Part model, mm, in its own coordinate system. Coordinates: 2 decimals unless noted, no trailing zeros. Order: outer loops, then holes, each group sorted by start corner. A loop starts at its lowest first (then second) coordinate and runs counter-clockwise, first axis right, second up. Notation, with made-up numbers: M -32.5,64 L -7.5,64 A6 ccw -7.5,73 Z; hole C 64,70.25 d4. An arc over 180 degrees is marked long. Answer in a Markdown table with one row per item. Add a question column.
from build123d import *

# Parameters (mm, degrees)
FILLET1_R          = 2.54
SKETCH2_R          = 1.395150395
CUT_EXTRUDE1_DEPTH = 126.080494205


with BuildPart() as part:
    # Sketch1 → Revolve1 (revolve)
    with BuildSketch(Plane.XY, mode=Mode.PRIVATE) as revolve1_sk:
        with BuildLine():
            Line((0, 76.2), (6.35, 76.2))
            Line((6.35, 76.2), (6.35, 63.5))
            ThreePointArc((6.35, 63.5), (51.251280605, 44.901280605), (69.85, 0))
            Line((69.85, 0), (63.5, 0))
            ThreePointArc((63.5, 0), (46.761152545, 40.411152545), (6.35, 57.15))
            Line((6.35, 57.15), (0, 57.15))
            Line((0, 57.15), (0, 76.2))
        make_face()
    revolve(revolve1_sk.sketch.rotate(Axis((0, 0, 0), (1, 0, 0)), 90), axis=Axis((0, 0, 0), (1, 0, 0)))

    # Fillet1
    fillet1_edges = [part.edges().sort_by_distance(p)[0] for p in [
        (6.35, 0, -63.5),
    ]]
    fillet(fillet1_edges, radius=FILLET1_R)

    # Sketch2 → Cut-Extrude1 (cut, through all)
    with BuildSketch(Plane(origin=(6.35, 0, 0), x_dir=(0, 0, -1), z_dir=(1, 0, 0))):
        with Locations((0, 73.025)):
            Circle(SKETCH2_R)
        with Locations((73.025, 0)):
            Circle(SKETCH2_R)
        with Locations((0, -73.025)):
            Circle(SKETCH2_R)
        with Locations((-73.025, 0)):
            Circle(SKETCH2_R)
    extrude(amount=-CUT_EXTRUDE1_DEPTH, mode=Mode.SUBTRACT)


solid = part.part
(1) Slice it at A-A (x = 57). List the corners of the cut face in (y, z).
(2) Wall check: line 1 (Y direction, x = 2.5, z = 0); line 2 (Y direction, x = 9.5, z = 42); line 3 (Y direction, x = 29, z = 32). Give the ranges that are in metal, low to high.
(3) Drop flat-ended pins along their axis: P1, Ø1.7, axis at y = 73.025, z = 0, coming from the -X side; P2, Ø8, axis at x = 15, z = 47, coming from the +Y side; P3, Ø3.5, axis at y = -73.025, z = 0, coming from the +X side; P4, Ø8, axis at x = 23.5, y = -0.5, coming from the +Z side. Give the stop position or say it passes through.
(4) Pull direction Y, two halves, no side cores. Call faces 1 (the cylindrical face through (3.219, 74.388, -16.519)), 2 (the cylindrical face through (3.131, -2.513, -57.095)), 3 (the flat face through (6.35, -57, -34)): pulls with the +Y half, pulls with the -Y half, needs draft (parallel to the pull), parting line crosses it, or undercut.
Computed:
| question | item | result |
|---|---|---|
| 1 | outline | C 0,0 d76.6; hole C 0,0 d52.94 |
| 2 | line 1 | y = -76.2 to -74.42, -71.63 to -57.15, 57.15 to 71.63, 74.42 to 76.2 |
| 2 | line 2 | y = -47.52 to -38.63, 38.63 to 47.52 |
| 2 | line 3 | y = -49.95 to -41.58, 41.58 to 49.95 |
| 3 | P1 | passes through |
| 3 | P2 | stops at y = 45.99 |
| 3 | P3 | stops at x = 6.35 |
| 3 | P4 | stops at z = 62.12 |
| 4 | face 1 | parting line crosses it |
| 4 | face 2 | undercut |
| 4 | face 3 | needs draft |
